Can you work these out from the model? Positions are in its coordinate system, mm. A direction names the side the tool comes from. Round coordinates to 2 decimals unless told otherwise and drop trailing zeros. Loops run counter-clockwise (first coordinate to the right, second up) from the corner with the lowest first, then second, coordinate; pieces in that order, holes last. Notation, with made-up numbers: (-32.5, 62.5) -> (9.5, 62.5) arc R25 cw to (9.5, 84.5) -> close; hole circle Ø4 at (64, 78.25). An arc over 180 degrees is marked (long way). Write item = value, one per line.
Autodesk Inventor part; units mm, degrees
ref_plane "Work Plane1" through (-14.235, 46, 0) normal (0, -1, 0) x (1, 0, 0)
ref_plane "YZ Plane" through (0, 0, 0) normal (1, 0, 0) x (0, 1, 0)
ref_plane "XZ Plane" through (0, 0, 0) normal (0, 1, 0) x (-1, 0, 0)
sketch "Sketch1" plane through (0, 0, 0) normal (0, 0, 1) x (1, 0, 0)
  line L0 (-9.235, 1) -> (9.235, 1)
  line L1 (11.235, 1.1946) -> (11.235, -1)
  line L2 (11.235, -1) -> (-11.235, -1)
  line L3 (-11.235, -1) -> (-11.235, 1.0973)
  line L4 (-9.235, 1) -> (-9.235, 13.5)
  line L5 (-9.235, 13.5) -> (-11.235, 13.5)
  line L6 (-11.235, 13.5) -> (-11.235, 1.0973)
  line L7 (9.235, 1) -> (9.235, 13.5)
  line L8 (9.235, 13.5) -> (11.235, 13.5)
  line L9 (11.235, 13.5) -> (11.235, 1.1946)
  line L10 (-14.235, -4) -> (14.065, -4)
  line L11 (14.065, -4) -> (14.065, 46)
  line L12 (14.065, 46) -> (-14.235, 46)
  line L13 (-14.235, 46) -> (-14.235, -4)
  arc A0 (14.065, 46) -> (-14.235, 46) centre (-0.085, 46) ccw
  point P0 (0, 0)
  point P1 (0, 0)
  dimension "d0" = 22.47
  dimension "d1" = 11.235
  dimension "d3" = 1
  dimension "d4" = 14.5
  dimension "d5" = 2
  dimension "d6" = 2
  dimension "d7" = 14.5
  dimension "d10" = 2
  dimension "d19" = 28.3
  dimension "d20" = 50
  dimension "d21" = 14.15
  dimension "d22" = 3
  dimension "d23" = 3
  dimension "d64" = 18.47
extrude "Extrusion2" add sketch "Sketch1" along normal blind 25
sketch "Sketch2" plane through (0, 0, 25) normal (0, 0, 1) x (1, 0, 0)
  line L0 (-14.235, 46) -> (-14.235, -4)
  line L1 (-14.235, -4) -> (14.065, -4)
  line L2 (14.065, -4) -> (14.065, 46)
  line L3 (14.065, -4) -> (14.065, 46)
  line L4 (-14.235, -4) -> (14.065, -4)
  line L5 (14.065, -4) -> (14.065, 46)
  line L6 (-14.235, 46) -> (-14.235, -4)
  arc A0 (14.065, 46) -> (-14.235, 46) centre (-0.085, 46) ccw
  point P0 (0, 0)
extrude "Extrusion3" add sketch "Sketch2" along normal blind 5
ref_plane "Work Plane1" through (-14.235, 46, 0) normal (0, -1, 0) x (1, 0, 0)
sketch "Sketch3" plane through (-14.235, 46, 0) normal (0, -1, 0) x (1, 0, 0)
  line L0 (0, 0) -> (28.3, 0)
  line L1 (28.3, 0) -> (28.3, 30)
  line L2 (0, 30) -> (28.3, 30)
  line L3 (0, 0) -> (0, 30)
  line L4 (14.235, 0) -> (42.81, 0) construction
  line L5 (28.3, 0) -> (28.3, 30)
  line L6 (31.8032, 0) -> (39.7036, -15.7866)
  line L7 (39.7036, -15.7866) -> (45.9635, -12.6539)
  line L8 (45.9635, -12.6539) -> (28.3, 22.6411)
  line L9 (28.3, 0) -> (0, 0)
  line L10 (28.3, 0) -> (31.8032, 0)
  line L11 (-3.5032, 0) -> (-11.4036, -15.7866)
  line L12 (-11.4036, -15.7866) -> (-17.6635, -12.6539)
  line L13 (-17.6635, -12.6539) -> (0, 22.6411)
  line L14 (0, 0) -> (-3.5032, 0)
  line L15 (0, 0) -> (0, 22.6411)
  dimension "d31" = 7
extrude "Extrusion4" add sketch "Sketch3" along normal blind 20 contours L14 L11 L12 L13 L3 | L1 L8 L7 L6 L10
sketch "Sketch4" plane through (0, 0, 0) normal (0, 0, -1) x (-1, 0, 0)
  line L0 (14.235, -4) -> (-14.065, -4)
  line L1 (0.085, -4) -> (0.085, 46)
  arc A0 (9.235, 46) -> (-9.065, 46) centre (0.085, 46) ccw
  line L2 (-9.065, 46) -> (-9.065, 21)
  line L3 (9.235, 46) -> (9.235, 21)
  arc A1 (14.235, 46) -> (-14.065, 46) centre (0.085, 46) ccw
  line L4 (-4.235, 21) -> (-4.235, 6)
  line L5 (-4.235, 6) -> (4.235, 6)
  line L6 (4.235, 6) -> (4.235, 21)
  line L7 (11.235, 13.5) -> (9.235, 13.5)
  line L8 (9.235, 13.5) -> (9.235, 1)
  line L9 (9.235, 1) -> (-9.235, 1)
  line L10 (-9.235, 1) -> (-9.235, 13.5)
  line L11 (-9.235, 13.5) -> (-11.235, 13.5)
  line L12 (-11.235, 13.5) -> (-11.235, -1)
  line L13 (-11.235, -1) -> (11.235, -1)
  line L14 (11.235, -1) -> (11.235, 13.5)
  line L15 (-9.065, 21) -> (-4.235, 21)
  line L16 (4.235, 21) -> (9.235, 21)
  point P0 (0, 0)
  dimension "d34" = 50
  dimension "d38" = 25
  dimension "d46" = 5
  dimension "d47" = 5
  dimension "d48" = 5
  dimension "d49" = 5
extrude "Extrusion5" cut sketch "Sketch4" against normal blind 30 contours L5 L4 L15 L2 A0 L3 L16 L6
chamfer "Chamfer1" distance 1 angle 45 6 edges at (-4.235, 21, 15) (4.235, 21, 15) (-4.235, 6, 15) (4.235, 6, 15) (9.065, 21, 15) (-9.235, 21, 15)
chamfer "Chamfer3" distance 1 angle 45 8 edges at (22.8967, 26, 4.9936) (28.5986, 26, -14.2202) (21.5184, 26, -7.8933) (15.8166, 26, 0) (-15.9866, 26, 0) (-21.6884, 26, -7.8933) (-28.7686, 26, -14.2202) (-23.0667, 26, 4.9936)
chamfer "Chamfer4" distance 1 angle 45 8 edges at (15.8166, 46, 0) (21.5184, 46, -7.8933) (22.8967, 46, 4.9936) (28.5986, 46, -14.2202) (-23.0667, 46, 4.9936) (-28.7686, 46, -14.2202) (-15.9866, 46, 0) (-21.6884, 46, -7.8933)
chamfer "Chamfer5" distance 1 angle 45 3 edges at (-0.085, 60.15, 30) (-14.235, 21, 30) (14.065, 21, 30)
equation "\"d6\" = d5"
equation "\"d7\" = d4"
equation "\"d10\" = d5"
properties part number "EndStopGeneric"
1. Suppose I cut it at B-B, the plane x = 19.5. List the corners of the cut face in (y, z) for me.
Entries:
outline = (26, -1.63) -> (27, -3.86) -> (45, -3.86) -> (46, -1.63) -> (46, 9.55) -> (45, 11.78) -> (27, 11.78) -> (26, 9.55) -> close
2. We'd pull the mould along X, two halves only. Please class faces 6 (the conical face through (-0.378, 59.32, 29.826)), 7 (the flat face through (0, 1, 12)), 8 (the flat face through (-23.19, 36.13, 4.75)), 9 (the flat face through (-21.63, 36.13, -7.78)): released by +X, released by -X, zero draft, split by the parting line, or undercut.
Entries:
face_6 = split by the parting line
face_7 = undercut
face_8 = released by -X
face_9 = undercut
3. Suppose I cut it at C-C, the plane y = 42. List the corners of the cut face in (x, z) for me (1 decimal).
Entries:
outline = (-31.9, -12.7) -> (-25.6, -15.8) -> (-17.7, 0) -> (-9.2, 0) -> (-9.2, 30) -> (-13.2, 30) -> (-14.2, 29) -> (-14.2, 22.6) -> close; (9.1, 0) -> (17.6, 0) -> (25.5, -15.8) -> (31.7, -12.7) -> (14.1, 22.6) -> (14.1, 29) -> (13.1, 30) -> (9.1, 30) -> close
4. Suppose I cut it at A-A, the plane y = 15. List the corners of the cut face in (x, z) for me (3 decimals).
Entries:
outline = (-14.235, 0) -> (-4.235, 0) -> (-4.235, 30) -> (-13.235, 30) -> (-14.235, 29) -> close; (4.235, 0) -> (14.065, 0) -> (14.065, 29) -> (13.065, 30) -> (4.235, 30) -> close
5. For faces 1 (the flat face through (4.235, 14, 15)), 2 (the flat face through (28.334, 26.507, -13.801)), 3 (the flat face through (-21, 26, 2)), 4 (the flat face through (21, 26, 0)), 5 (the flat face through (10, 13.5, 12)), which set-ups out of +Z, -Z, +X, -X, +Y, -Y let a thin tool reach every point of the face, with its end or its side?
Entries:
face_1 = +Z, -Z
face_2 = -Z, +X, -Y
face_3 = +Z, -Z, -X, -Y
face_4 = +Z, -Z, +X, -Y
face_5 = -Z
6. Suppose I cut it at D-D, the plane z = -7. List the corners of the cut face in (x, y) for me, and give its area (3 significant figures).
Entries:
outline = (-29.07, 27) -> (-27.95, 26) -> (-22.36, 26) -> (-21.24, 27) -> (-21.24, 45) -> (-22.36, 46) -> (-27.95, 46) -> (-29.07, 45) -> close; (21.07, 27) -> (22.19, 26) -> (27.78, 26) -> (28.9, 27) -> (28.9, 45) -> (27.78, 46) -> (22.19, 46) -> (21.07, 45) -> close
area = 309 mm²
7. I'm going to push flat-ended pins straight in: pin 1 (12 mm diameter, centred on y = 32.5, z = 10, fed in from -X); pin 2 (4 mm diameter, centred on x = 7.5, y = 52.5, fed in from -Z); pin 3 (3 mm diameter, centred on y = 30, z = 24.5, fed in from +X) (3 decimals); pin 4 (11 mm diameter, centred on x = 0.5, z = 12, fed in from +Y). Where does each tip first touch, or does it pass through?
Entries:
pin_1 = -23.56
pin_2 = 0
pin_3 = 14.065
pin_4 = 60.15
8. I need wall thicknesses on line 1 (X direction, y = 17, z = 11) (3 decimals); line 2 (X direction, y = 24, z = 26.5) (3 decimals); line 3 (Y direction, x = -4.5, z = 23) (3 decimals). Which ranges of each line are inside material? Lowest first, please. Write a range as [from, to].
Entries:
line_1 = [-14.235, -4.235], [4.235, 14.065]
line_2 = [-14.235, -9.235], [9.065, 14.065]
line_3 = [-4, -1], [1, 20.265], [54.014, 59.444]
